from build123d import *

# Parameters (mm, degrees)
SKETCH_1_R          = 25
EXTRUDE_1_DEPTH     = 50
SKETCH_2_R          = 20
CUT_EXTRUDE_1_DEPTH = 48
EXTRUDE_2_DEPTH     = 18
SKETCH_4_OUTSIDE_W  = 101.712
SKETCH_4_OUTSIDE_H  = 102.234
SKETCH_4_OUTSIDE_R  = 27
CUT_EXTRUDE_3_DEPTH = 10
CUT_EXTRUDE_3_DRAFT = -45
SKETCH_5_OUTSIDE_W  = 101.712
SKETCH_5_OUTSIDE_H  = 102.234
SKETCH_5_OUTSIDE_R  = 27
CUT_EXTRUDE_4_DEPTH = 10
CUT_EXTRUDE_4_DRAFT = -45
SKETCH_6_R          = 22.55
SKETCH_6_R_2        = 19.55
EXTRUDE_1_2_DEPTH   = 29.325
FILLET_1_R          = 1.666666667
CHAMFER_1_SIZE      = 1.303333333
FILLET_2_R          = 1.303333333


with BuildPart() as part:
    # Эскиз1 → Extrude 1 (new body)
    with BuildSketch(Plane(origin=(0, 0, 0), x_dir=(0, 0, -1), z_dir=(1, 0, 0))):
        Circle(SKETCH_1_R)
    extrude(amount=-EXTRUDE_1_DEPTH)

    # Эскиз2 → Вырез-Вытянуть1 (cut)
    with BuildSketch(Plane.ZY.offset(50)):
        Circle(SKETCH_2_R)
    extrude(amount=-CUT_EXTRUDE_1_DEPTH, mode=Mode.SUBTRACT)

    # Эскиз3 → Бобышка-Вытянуть2 (add)
    with BuildSketch(Plane(origin=(0, 0, 0), x_dir=(0, 0, -1), z_dir=(1, 0, 0))):
        Polygon((22.398442547, -21.686626558), (29.980390795, 8.554306971), (7.581948249, 30.24093353), (-22.398442547, 21.686626558), (-29.980390795, -8.554306971), (-7.581948249, -30.24093353), align=None)
    extrude(amount=-EXTRUDE_2_DEPTH)


with BuildPart() as cut_extrude_3_tool:
    # Эскиз4 outside → Вырез-Вытянуть3 (with draft: the straight prism first)
    with BuildSketch(Plane(origin=(0, 0, 0), x_dir=(0, 0, -1), z_dir=(1, 0, 0))):
        Rectangle(SKETCH_4_OUTSIDE_W, SKETCH_4_OUTSIDE_H)
        Circle(SKETCH_4_OUTSIDE_R, mode=Mode.SUBTRACT)
    extrude(amount=-CUT_EXTRUDE_3_DEPTH)
    # Вырез-Вытянуть3: the draft: its side faces are tilted about the plane it starts from
    cut_extrude_3_sides = [cut_extrude_3_tool.faces().sort_by_distance(p)[0] for p in [
        (-5, -51.117, 0),
        (-5, 0, -50.856),
        (-5, 51.117, 0),
        (-5, 0, 50.856),
        (-5, 0, 27),
    ]]
    draft(cut_extrude_3_sides, Plane(origin=(0, 0, 0), x_dir=(0, 0, -1), z_dir=(1, 0, 0)), CUT_EXTRUDE_3_DRAFT)


with BuildPart() as part_1:
    add(part.part)

    # Вырез-Вытянуть3: cut by cut_extrude_3_tool
    add(cut_extrude_3_tool.part, mode=Mode.SUBTRACT)


with BuildPart() as cut_extrude_4_tool:
    # Эскиз5 outside → Вырез-Вытянуть4 (with draft: the straight prism first)
    with BuildSketch(Plane.ZY.offset(18)):
        Rectangle(SKETCH_5_OUTSIDE_W, SKETCH_5_OUTSIDE_H)
        Circle(SKETCH_5_OUTSIDE_R, mode=Mode.SUBTRACT)
    extrude(amount=-CUT_EXTRUDE_4_DEPTH)
    # Вырез-Вытянуть4: the draft: its side faces are tilted about the plane it starts from
    cut_extrude_4_sides = [cut_extrude_4_tool.faces().sort_by_distance(p)[0] for p in [
        (-13, -51.117, 0),
        (-13, 0, 50.856),
        (-13, 51.117, 0),
        (-13, 0, -50.856),
        (-13, 0, -27),
    ]]
    draft(cut_extrude_4_sides, Plane.ZY.offset(18), CUT_EXTRUDE_4_DRAFT)


with BuildPart() as part_2:
    add(part_1.part)

    # Вырез-Вытянуть4: cut by cut_extrude_4_tool
    add(cut_extrude_4_tool.part, mode=Mode.SUBTRACT)

    # Эскиз6 → Extrude 1 2 (add)
    with BuildSketch(Plane(origin=(0, 0, 0), x_dir=(0, 0, -1), z_dir=(1, 0, 0))):
        Circle(SKETCH_6_R)
        Circle(SKETCH_6_R_2, mode=Mode.SUBTRACT)
    extrude(amount=EXTRUDE_1_2_DEPTH)

    # Скругление1
    fillet_1_edges = [part_2.edges().sort_by_distance(p)[0] for p in [
        (-50, 0, 25),
        (-50, 0, -20),
    ]]
    fillet(fillet_1_edges, radius=FILLET_1_R)

    # Фаска1
    chamfer_1_edges = [part_2.edges().sort_by_distance(p)[0] for p in [
        (29.325, 0, 19.55),
    ]]
    chamfer(chamfer_1_edges, length=CHAMFER_1_SIZE)

    # Скругление2
    fillet_2_edges = [part_2.edges().sort_by_distance(p)[0] for p in [
        (29.325, 0, 22.55),
    ]]
    fillet(fillet_2_edges, radius=FILLET_2_R)


solid = part_2.part
Work out the finished part from the listing and answer in its coordinate system (mm). A direction names the side the tool comes from. Round coordinates to 2 decimals unless told otherwise and drop trailing zeros. Loops run counter-clockwise (first coordinate to the right, second up) from the corner with the lowest first, then second, coordinate; pieces in that order, holes last. Notation, with made-up numbers: (3, 74) - (50, 74) arc R8 ccw to (50, 80) - close; hole circle Ø7 at (-35.75, 51). An arc over 180 degrees is marked (long way). One line per item, written item: value.
Q1. Find section A-A on x = 17. Give the vertices of the cut face in (y, z), and give its area (3 significant figures).
Check values:
outline: circle Ø45.1 at (0, 0); hole circle Ø39.1 at (0, 0)
area: 397 mm2
Q2. Straight lines are drawn through the part: probe 1 along Y at (x, z) = (-31, 0); probe 2 along Z at (x, y) = (-41, -15.5); probe 3 along Z at (x, y) = (-29, 9). For each, find the intervals that lie inside material, in ascending order.
Check values:
probe 1: -25 to -20, 20 to 25
probe 2: -19.62 to -12.64, 12.64 to 19.62
probe 3: -23.32 to -17.86, 17.86 to 23.32
Q3. Each of these flat-tipped pins is pushed along its axis until it touches: pin 1 Ø2 at (x, y) = (-9, 16) entering from +Z; pin 2 Ø3 at (y, z) = (8.5, 0.5) entering from +X; pin 3 Ø3 at (x, y) = (-21.5, -18.5) entering from -Z; pin 4 Ø1 at (y, z) = (20.5, -18.5) entering from -X. Where does it stop, or does it pass through?
Check values:
pin 1: z = 24.07
pin 2: x = 0
pin 3: z = -18.33
pin 4: through
Q4. The mould has two halves that part along Y. Classify faces 1 (the flat face through (-8.874, -26.024, -7.198)), 2 (the flat face through (0, 0, 0)), 3 (the flat face through (-8.874, 6.778, 26.136)): +Y half, -Y half, draft (parallel to the pull), parting line (faces both ways), or undercut.
Check values:
face 1: -Y half
face 2: undercut
face 3: +Y half
Q5. For faces 4 (the conical face through (-0.996, 19.523, 20.065)), 5 (the cylindrical face through (13.815, 19.014, -12.123)), 6 (the cylindrical face through (-32.954, 7.509, -23.846)), determine the directions among +Z, -Z, +X, -X, +Y, -Y from which every point of the face is accessible in a straight line to the end or side of a thin tool.
Check values:
face 4: +Z, +X, +Y
face 5: +X
face 6: -X
Q6. Find section B-B on x = -6.5. Give the vertices of the cut face in (y, z).
Check values:
outline: (-30.24, 7.58) - (-21.69, -22.4) - (8.55, -29.98) - (30.24, -7.58) - (21.69, 22.4) - (-8.55, 29.98) - close
